The model under review builds one solid part; all positions refer to its coordinate system, in mm. A direction names the side the tool comes from. Coordinates: 2 decimals unless noted, no trailing zeros. Order: outer loops, then holes, each group sorted by start corner. A loop starts at its lowest first (then second) coordinate and runs counter-clockwise, first axis right, second up.
from build123d import *

# Parameters (mm, degrees)
F1_DEPTH = 4.7625


with BuildPart() as f1:
    # F0 (on Right) → F1 (new body, symmetric)
    with BuildSketch(Plane.YZ):
        with BuildLine():
            Line((178.64784, -78.256549), (178.64784, 74.143451))
            Line((178.64784, 74.143451), (-89.029852, 42.679582))
            ThreePointArc((-89.029852, 42.679582), (-93.675787, 41.189865), (-97.417243, 38.058494))
            ThreePointArc((-97.417243, 38.058494), (-119.633425, 23.324748), (-146.283933, 23.951184))
            ThreePointArc((-146.283933, 23.951184), (-164.555034, 28.926971), (-183.30216, 31.598451))
            Line((-183.30216, 31.598451), (-180.33696, 6.372124))
            Line((-180.33696, 6.372124), (-291.243161, -6.664219))
            ThreePointArc((-291.243161, -6.664219), (-296.612067, -11.242249), (-294.43711, -17.954406))
            Line((-294.43711, -17.954406), (-287.389228, -23.519688))
            ThreePointArc((-287.389228, -23.519688), (-285.182532, -24.646288), (-282.71268, -24.842665))
            Line((-282.71268, -24.842665), (-187.686579, -13.67293))
            ThreePointArc((-187.686579, -13.67293), (-176.18102, -13.63024), (-164.959982, -16.173468))
            ThreePointArc((-164.959982, -16.173468), (-125.920012, -40.965213), (-101.91306, -80.492622))
            Line((-101.91306, -80.492622), (-54.8202, -61.442622))
            ThreePointArc((-54.8202, -61.442622), (-55.877698, -59.54941), (-56.543876, -57.485735))
            ThreePointArc((-56.543876, -57.485735), (-53.806121, -47.605216), (-44.114969, -44.258345))
            Line((-44.114969, -44.258345), (178.64784, -78.256549))
        make_face()
    extrude(amount=F1_DEPTH, both=True)


solid = f1.part
(1) Wall thickness on line 1 (Y direction, x = 1, z = -40.5); line 2 (Z direction, x = 0.25, y = -41.5); line 3 (Z direction, x = -1.25, y = 145): over which ranges is each line inside the solid? List them lowest first.
(2) The part is to be moulded in two halves that separate along Y. For faces 1 (the face through (0.067, -164.295, 28.873)), 2 (the face through (-4.762, -10, -2)), 3 (the face through (0, 178.648, -3)), 4 (the face through (0.07, -93.62, 41.22)), say which applies: +Y half, -Y half, draft (parallel to the pull), parting line (faces both ways), or undercut.
(3) Insertion check: pin 1 Ø3 at (x, z) = (-3, -62.5) entering from -Y; pin 2 Ø3 at (x, z) = (-3.5, -42.5) entering from -Y; pin 3 Ø1 at (x, z) = (3.5, 38.5) entering from -Y. Each pin has a flat end and moves straight along its axis. Give the tip position at first contact, or say it passes through.
(4) Consider section A-A (z = -70). Give the boundary of the cut face in (x, y), then the cut area to 3 significant figures.
(5) Consider section B-B (x = -2.5). Give the boundary of the cut face in (y, z), then the cut area to 3 significant figures.
(6) Tool access review of faces 5 (the face through (0.07, 46.68, 58.63)), 6 (the face through (0.067, -78.696, -71.101)), 7 (the face through (0.07, -181.84, 19.16)): name each direction out of +Z, -Z, +X, -X, +Y, -Y from which nothing blocks a thin tool from reaching the whole face with its end or side.
(7) Consider section D-D (y = -6). Give the boundary of the cut face in (x, z), then the cut area to 3 significant figures.
(8) Consider section C-C (z = -48.5). Give the boundary of the cut face in (x, y).
Findings:
1. line 1: y = -126.38 to 178.65
1. line 2: z = -44.66 to 48.27
1. line 3: z = -73.12 to 70.19
2. face 1: undercut
2. face 2: draft
2. face 3: +Y half
2. face 4: -Y half
3. pin 1: stops at y = -110.65
3. pin 2: stops at y = -125.89
3. pin 3: stops at y = -97.46
4. outline: (-4.76, -106) - (4.76, -106) - (4.76, -75.97) - (-4.76, -75.97) - close; (-4.76, 124.55) - (4.76, 124.55) - (4.76, 178.65) - (-4.76, 178.65) - close
4. area: 801 mm2
5. outline: (-294.44, -17.95) - (-287.39, -23.52) arc R6.35 ccw to (-282.71, -24.84) - (-187.69, -13.67) arc R50.89 cw to (-164.96, -16.17) arc R101.6 cw to (-101.91, -80.49) - (-54.82, -61.44) arc R11.02 cw to (-56.54, -57.49) arc R11.02 cw to (-44.11, -44.26) - (178.65, -78.26) - (178.65, 74.14) - (-89.03, 42.68) arc R12.7 ccw to (-97.42, 38.06) arc R44.45 cw to (-146.28, 23.95) arc R152.4 ccw to (-183.3, 31.6) - (-180.34, 6.37) - (-291.24, -6.66) arc R6.35 ccw to start
5. area: 40,500 mm2
6. face 5: +Z, +X, -X, -Y
6. face 6: -Z, +X, -X
6. face 7: +X, -X, -Y
7. outline: (-4.76, -50.08) - (4.76, -50.08) - (4.76, 52.44) - (-4.76, 52.44) - close
7. area: 976 mm2
8. outline: (-4.76, -119.23) - (4.76, -119.23) - (4.76, -54.56) - (-4.76, -54.56) - close; (-4.76, -16.32) - (4.76, -16.32) - (4.76, 178.65) - (-4.76, 178.65) - close
